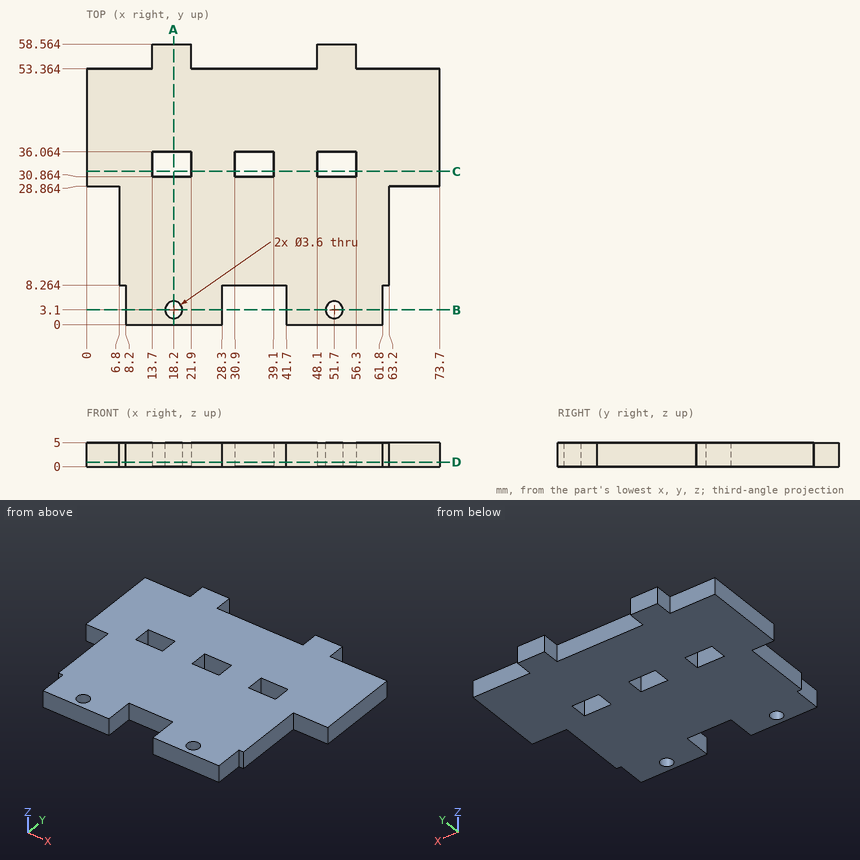
Here's the drawing with two shaded views (mm, measured from the low corner). I have some questions. Give positions to 0.01 mm unless a question says otherwise; leave off trailing zeros. Write each loop counter-clockwise with the first axis right and the second up, starting at its lowest first coordinate (ties: lowest second). Pieces come first, ordered by that corner, then holes. Notation, with made-up numbers: (-20.75, -2) -> (30.25, -2) arc R9 cw to (30.25, 10) -> close; hole circle Ø9 at (26, 65.25). An arc over 180 degrees is marked (long way). Answer as a JSON object with one key per item and string values. Group by question number.
Item 1: Suppose I cut it at A-A (x = 18.2). Please give me the cut outline in (y, z), plus the area to 3 significant figures.
Item 2: I'm going to push flat-ended pins straight in: P1, Ø2.5, axis at x = 37, z = 2, coming from the -Y side; P2, Ø2.5, axis at y = 55.5, z = 2.5, coming from the +X side; P3, Ø2.5, axis at y = 56.5, z = 3.5, coming from the -X side. Where does each tip first touch, or does it pass through?
Item 3: Suppose I cut it at C-C (y = 32). Please give me the cut outline in (x, z).
Item 4: Suppose I cut it at B-B (y = 3.1). Please give me the cut outline in (x, z).
Item 5: Suppose I cut it at D-D (z = 0.95). State how many separate pieces and enclosed holes the cut face has, plus the area to 3 significant figures.
Item 6: Please list where these lines run through material, in increasing order: line 1 (X direction, y = 35.5, z = 3.2); line 2 (X direction, y = 3, z = 3.15); line 3 (Y direction, x = 18.2, z = 2). Write a range as [from, to].
Findings:
{
 "1": {"outline": "(0, 0) -> (1.3, 0) -> (1.3, 5) -> (0, 5) -> close; (4.9, 0) -> (30.86, 0) -> (30.86, 5) -> (4.9, 5) -> close; (36.06, 0) -> (58.56, 0) -> (58.56, 5) -> (36.06, 5) -> close", "area": "249 mm²"},
 "2": {"P1": "stops at y = 8.26", "P2": "stops at x = 56.3", "P3": "stops at x = 13.7"},
 "3": {"outline": "(0, 0) -> (13.7, 0) -> (13.7, 5) -> (0, 5) -> close; (21.9, 0) -> (30.9, 0) -> (30.9, 5) -> (21.9, 5) -> close; (39.1, 0) -> (48.1, 0) -> (48.1, 5) -> (39.1, 5) -> close; (56.3, 0) -> (73.7, 0) -> (73.7, 5) -> (56.3, 5) -> close"},
 "4": {"outline": "(8.2, 0) -> (16.4, 0) -> (16.4, 5) -> (8.2, 5) -> close; (20, 0) -> (28.3, 0) -> (28.3, 5) -> (20, 5) -> close; (41.7, 0) -> (49.9, 0) -> (49.9, 5) -> (41.7, 5) -> close; (53.5, 0) -> (61.8, 0) -> (61.8, 5) -> (53.5, 5) -> close"},
 "5": {"separate pieces": "1", "enclosed holes": "5", "area": "3,240 mm²"},
 "6": {"line 1": "x = [0, 13.7], [21.9, 30.9], [39.1, 48.1], [56.3, 73.7]", "line 2": "x = [8.2, 16.4], [20, 28.3], [41.7, 49.9], [53.5, 61.8]", "line 3": "y = [0, 1.3], [4.9, 30.86], [36.06, 58.56]"}
}
